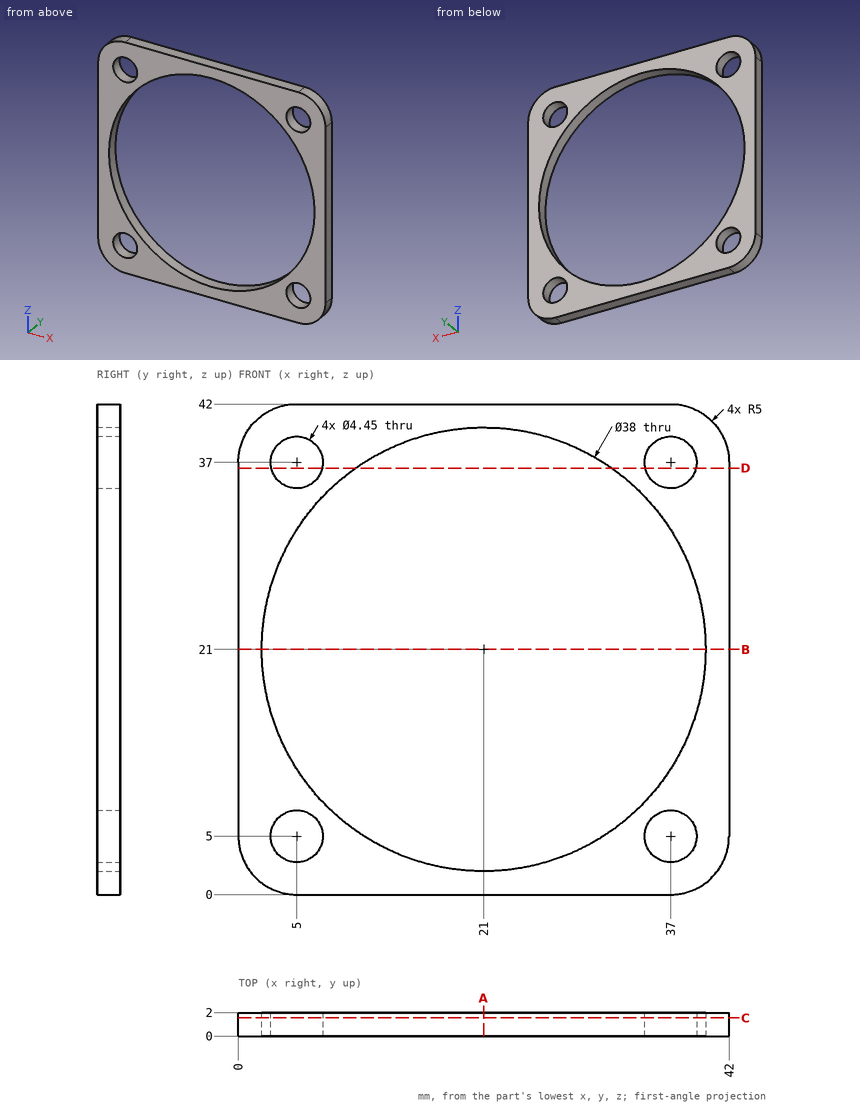
Here's the drawing with two shaded views (mm, measured from the low corner). I have some questions. Round coordinates to 2 decimals unless told otherwise and drop trailing zeros. Write each loop counter-clockwise with the first axis right and the second up, starting at its lowest first coordinate (ties: lowest second). Pieces come first, ordered by that corner, then holes.
(1) Suppose I cut it at D-D on z = 36.5. Write out the boundary of the cut face in (x, y), and give its area (3 significant figures).
Findings below:
outline: (0, 0) - (2.83, 0) - (2.83, 2) - (0, 2) - close; (7.17, 0) - (10.01, 0) - (10.01, 2) - (7.17, 2) - close; (31.99, 0) - (34.83, 0) - (34.83, 2) - (31.99, 2) - close; (39.17, 0) - (42, 0) - (42, 2) - (39.17, 2) - close
area: 22.7 mm2
(2) If I drill on probe 1 along Z at (x, y) = (21, 1.5); probe 2 along Z at (x, y) = (4.5, 1); probe 3 along Z at (x, y) = (5, 1) (3 decimals), over which ranges is the centre line in solid material (lowest first)?
Findings below:
probe 1: z = 0 to 2, 40 to 42
probe 2: z = 0.03 to 2.83, 7.17 to 11.58, 30.42 to 34.83, 39.17 to 41.97
probe 3: z = 0 to 2.775, 7.225 to 10.753, 31.247 to 34.775, 39.225 to 42
(3) Suppose I cut it at A-A on x = 21. Write out the boundary of the cut face in (y, z), and give its area (3 significant figures).
Findings below:
outline: (0, 0) - (2, 0) - (2, 2) - (0, 2) - close; (0, 40) - (2, 40) - (2, 42) - (0, 42) - close
area: 8.00 mm2
(4) Suppose I cut it at B-B on z = 21. Write out the boundary of the cut face in (x, y), and give its area (3 significant figures).
Findings below:
outline: (0, 0) - (2, 0) - (2, 2) - (0, 2) - close; (40, 0) - (42, 0) - (42, 2) - (40, 2) - close
area: 8.00 mm2
(5) Suppose I cut it at C-C on y = 1.55. Write out the boundary of the cut face in (x, z) (3 decimals), and give its area (3 significant figures).
Findings below:
outline: (0, 5) arc R5 ccw to (5, 0) - (37, 0) arc R5 ccw to (42, 5) - (42, 37) arc R5 ccw to (37, 42) - (5, 42) arc R5 ccw to (0, 37) - close; hole circle Ø38 at (21, 21); hole circle Ø4.45 at (5, 5); hole circle Ø4.45 at (5, 37); hole circle Ø4.45 at (37, 5); hole circle Ø4.45 at (37, 37)
area: 546 mm2
(6) For pin 1 (3.5 mm diameter, centred on x = 37, z = 37, fed in from -Y), with a flat end and sliding along its axis, tell me the tip position at first contact or that it passes through.
Findings below:
pin 1: passes through
